Can you work these out from the model? Positions are in its coordinate system, mm. A direction names the side the tool comes from. Give positions to 0.01 mm unless a question says otherwise; leave off trailing zeros. Write each question's results on one line, items separated by ' | '. Start each with the question number.
from build123d import *

# Parameters (mm, degrees)
BOSS_EXTRUDE1_DEPTH     = 6
CUT_EXTRUDE1_DEPTH      = 164.636793074
CUT_EXTRUDE1_DEPTH_BACK = 164.636793074
SKETCH2_R               = 1.75
BOSS_EXTRUDE2_DEPTH     = 20
SKETCH4_W               = 132.33663358
SKETCH4_H               = 54.683142632
CUT_EXTRUDE2_DEPTH      = 20


with BuildPart() as part:
    # Sketch1 → Boss-Extrude1 (new body)
    with BuildSketch(Plane(origin=(0, 0, 0), x_dir=(1, 0, 0), z_dir=(0, 1, 0))):
        with BuildLine():
            Line((0, 0), (-121, 0))
            Line((-121, 0), (-121, -30.298554482))
            add(Edge.make_bspline(
                [(-121, -30.298554482), (-89.558533356, -59.655086777), (-53.189409509, -82.739680225), (-20.07, -110)],
                knots=[0, 0, 0, 0, 1, 1, 1, 1], degree=3))
            Line((-20.07, -110), (0, -110))
            Line((0, -110), (0, 0))
        make_face()
    extrude(amount=BOSS_EXTRUDE1_DEPTH)

    # Sketch2 → Cut-Extrude1 (cut, two sides: drawn at the far end of the back side and taken through both)
    with BuildSketch(Plane(origin=(0, 0, 0), x_dir=(-1, 0, 0), z_dir=(0, 0, -1)).offset(-CUT_EXTRUDE1_DEPTH_BACK)):
        with Locations((3, 3)):
            Circle(SKETCH2_R)
    extrude(amount=CUT_EXTRUDE1_DEPTH + CUT_EXTRUDE1_DEPTH_BACK, mode=Mode.SUBTRACT)

    # Sketch3 → Boss-Extrude2 (add)
    with BuildSketch(Plane(origin=(0, 6, 0), x_dir=(1, 0, 0), z_dir=(0, 1, 0))):
        with BuildLine():
            Line((-118, -3), (-118, 0))
            Line((-118, 0), (-121, 0))
            Line((-121, 0), (-121, -30.298554482))
            add(Edge.make_bspline(
                [(-121, -30.298554482), (-89.558533356, -59.655086777), (-53.189409509, -82.739680225), (-20.07, -110)],
                knots=[0, 0, 0, 0, 1, 1, 1, 1], degree=3))
            Line((-20.07, -110), (-18.995872781, -110))
            Line((-18.995872781, -110), (-18.995872781, -107))
            add(Edge.make_bspline(
                [(-118, -28.991909602), (-110.289824181, -36.137206416), (-102.272955066, -42.924098905), (-85.87961507, -56.077650281), (-77.513636875, -62.436539609), (-52.27420649, -81.325206417), (-35.258396574, -93.669770918), (-18.995872781, -107)],
                knots=[0, 0, 0, 0, 0.25, 0.25, 0.5, 0.5, 1, 1, 1, 1], degree=3))
            Line((-118, -28.991909602), (-118, -3))
        make_face()
        Polygon((-3, -3), (-3, 0), (0, 0), (0, -110), (-3, -110), (-3, -107), align=None)
    extrude(amount=BOSS_EXTRUDE2_DEPTH)

    # Sketch4 → Cut-Extrude2 (cut)
    with BuildSketch(Plane(origin=(0, 4.5, 2.598076211), x_dir=(-1, 0, 0), z_dir=(0, -0.8660254037844398, -0.499999999999998))):
        with Locations((60.84284102, -6.354682021)):
            Rectangle(SKETCH4_W, SKETCH4_H)
    extrude(amount=CUT_EXTRUDE2_DEPTH, mode=Mode.SUBTRACT)


solid = part.part
Q1. Will these pins go through, and if not, where does the flat tip stop? P1, Ø1, axis at x = -39.5, y = 22.5, coming from the -Z side; P2, Ø8, axis at x = -94, y = 11, coming from the +Z side; P3, Ø6, axis at x = -70.5, y = 15.5, coming from the +Z side.
Q2. If I drill on probe 1 along Y at (x, z) = (-50, 57); probe 2 along X at (y, z) = (9, 11); probe 3 along X at (y, z) = (3, 72), over which ranges is the centre line in solid material (lowest first)? Write a range as from..to.
Q3. Which directions (+Z, -Z, +X, -X, +Y, -Y) give clear straight access to the entire face, cutting with the end or side of a thin tool? Please do faces 1 (the flat face through (-118, 16, 15)), 2 (the flat face through (-3, 16, 54)), 3 (the flat face through (-121, 13, 15)).
Q4. Thinking about a two-plate mould opening in X: for faces 4 (the flat face through (0, 13, 56)), 5 (the flat face through (-18.996, 16, 109)), 6 (the flat face through (-1, 26, 54)), which applies, released by +X, released by -X, zero draft, split by the parting line, or undercut?
Findings below:
1) P1: stops at z = 90.49 | P2: stops at z = 56.56 | P3: stops at z = 73.67
2) probe 1: y = 0..6 | probe 2: x = -121..-118, -3..0 | probe 3: x = -69.74..-4.75, -1.25..0
3) face 1: -Z, +Y | face 2: +Z, -Z, +Y | face 3: +Z, -Z, -X, +Y, -Y
4) face 4: released by +X | face 5: undercut | face 6: zero draft
